Work out the finished part from the listing and answer in its coordinate system (mm). Coordinates: 2 decimals unless noted, no trailing zeros. Write each loop counter-clockwise with the first axis right and the second up, starting at its lowest first coordinate (ties: lowest second). Pieces come first, ordered by that corner, then holes. Notation, with made-up numbers: (45.25, 9) - (101.25, 9) arc R29 ccw to (101.25, 47) - close; hole circle Ø4 at (3, 52.25). An arc over 180 degrees is marked (long way). Use a Markdown table: item, result. Add a question column.
(1) Given pin 1 Ø7 at (x, y) = (-124.636, 30) entering from +Z; pin 2 Ø9 at (x, y) = (123.364, 90) entering from +Z, each flat-ended and moving along its own axis, determine where each tip first touches the part or whether it passes through.
(2) For a pull along Y with two mould halves and no side action, classify faces 1 (the face through (-32.157, -123.966, 151.736)), 2 (the face through (-120, 10, 150.75)), 3 (the face through (-120.94, 1.53, 151.74)) as released by +Y, released by -Y, zero draft, split by the parting line, or undercut.
(3) The part is cut by section B-B, the plane x = -108. Give the vertices of the cut face in (y, z), then the cut area to 3 significant figures.
(4) The part is cut by section C-C, the plane y = 83. Give the vertices of the cut face in (x, z).
(5) Find the intervals of material crossed by line 1 (X direction, y = -19, z = 152.15); line 2 (Y direction, x = 48, z = 151.7); line 3 (X direction, y = 89, z = 152.3), in increasing order. Write a range as from..to.
(6) The part is cut by section A-A, the plane y = 0. Give the vertices of the cut face in (x, z).
(7) The part is cut by section D-D, the plane z = 151.7. State how many separate pieces and enclosed holes the cut face has, then the cut area to 3 significant figures.
Autodesk Inventor part; units mm, degrees
ref_plane "YZ Plane" through (0, 0, 0) normal (1, 0, 0) x (0, 1, 0)
ref_plane "XZ Plane" through (0, 0, 0) normal (0, 1, 0) x (-1, 0, 0)
ref_plane "XY Plane" through (0, 0, 0) normal (0, 0, 1) x (1, 0, 0)
ref_plane "РабПлоскость1" through (-270.6167, -11.8042, 150.75) normal (0, 0, 1) x (1, 0, 0)
sketch "Эскиз1" plane through (-270.6167, -11.8042, 150.75) normal (0, 0, 1) x (1, 0, 0)
  circle A0 centre (393.9807, -108.1958) radius 4
  circle A1 centre (393.9807, -78.1958) radius 4
  circle A2 centre (393.9807, -48.1958) radius 4
  circle A3 centre (393.9807, -18.1958) radius 4
  circle A4 centre (393.9807, 11.8042) radius 4
  circle A5 centre (393.9807, 41.8042) radius 4
  circle A6 centre (393.9807, 71.8042) radius 4
  circle A7 centre (393.9807, 101.8042) radius 4
  circle A8 centre (393.9807, 131.8042) radius 4
  circle A9 centre (362.9807, -108.1958) radius 4
  circle A10 centre (362.9807, 131.8042) radius 4
  circle A11 centre (331.9807, -108.1958) radius 4
  circle A12 centre (331.9807, 131.8042) radius 4
  circle A13 centre (300.9807, -108.1958) radius 4
  circle A14 centre (300.9807, 131.8042) radius 4
  circle A15 centre (269.9807, -108.1958) radius 4
  circle A16 centre (269.9807, 131.8042) radius 4
  circle A17 centre (238.9807, -108.1958) radius 4
  circle A18 centre (238.9807, 131.8042) radius 4
  circle A19 centre (207.9807, -108.1958) radius 4
  circle A20 centre (207.9807, 131.8042) radius 4
  circle A21 centre (176.9807, -108.1958) radius 4
  circle A22 centre (176.9807, 131.8042) radius 4
  circle A23 centre (145.9807, -108.1958) radius 4
  circle A24 centre (145.9807, -78.1958) radius 4
  circle A25 centre (145.9807, -48.1958) radius 4
  circle A26 centre (145.9807, -18.1958) radius 4
  circle A27 centre (145.9807, 11.8042) radius 4
  circle A28 centre (145.9807, 41.8042) radius 4
  circle A29 centre (145.9807, 71.8042) radius 4
  circle A30 centre (145.9807, 101.8042) radius 4
  circle A31 centre (145.9807, 131.8042) radius 4
  line L0 (385.9807, 121.8042) -> (385.9807, -98.1958)
  line L1 (385.9807, -98.1958) -> (155.9807, -98.1958)
  line L2 (155.9807, -98.1958) -> (155.9807, 121.8042)
  line L3 (155.9807, 121.8042) -> (385.9807, 121.8042)
  arc A32 (137.9807, 141.8042) -> (135.9807, 139.8042) centre (137.9807, 139.8042) ccw
  line L4 (135.9807, 139.8042) -> (135.9807, -116.1958)
  arc A33 (135.9807, -116.1958) -> (137.9807, -118.1958) centre (137.9807, -116.1958) ccw
  line L5 (137.9807, -118.1958) -> (403.2527, -118.1958)
  arc A34 (403.2527, -118.1958) -> (405.2527, -116.1958) centre (403.2527, -116.1958) ccw
  line L6 (405.2527, -116.1958) -> (405.2527, 139.8042)
  arc A35 (405.2527, 139.8042) -> (403.2527, 141.8042) centre (403.2527, 139.8042) ccw
  line L7 (403.2527, 141.8042) -> (137.9807, 141.8042)
  point P0 (270.6167, 11.8042)
extrude "Выдавливание1" add sketch "Эскиз1" along normal blind 2
properties part number "Прокладка рубашки охлаждения"
Model answer:
| question | item | result |
|---|---|---|
| 1 | pin 1 | through |
| 1 | pin 2 | z = 152.75 |
| 2 | face 1 | undercut |
| 2 | face 2 | zero draft |
| 2 | face 3 | undercut |
| 3 | outline | (-130, 150.75) - (-110, 150.75) - (-110, 152.75) - (-130, 152.75) - close; (110, 150.75) - (130, 150.75) - (130, 152.75) - (110, 152.75) - close |
| 3 | area | 80.0 mm^2 |
| 4 | outline | (-134.64, 150.75) - (-114.64, 150.75) - (-114.64, 152.75) - (-134.64, 152.75) - close; (115.36, 150.75) - (134.64, 150.75) - (134.64, 152.75) - (115.36, 152.75) - close |
| 5 | line 1 | -134.64..-114.64, 115.36..134.64 |
| 5 | line 2 | -130..-110, 110..130 |
| 5 | line 3 | -134.64..-128.51, -120.76..-114.64, 115.36..119.49, 127.24..134.64 |
| 6 | outline | (-134.64, 150.75) - (-128.64, 150.75) - (-128.64, 152.75) - (-134.64, 152.75) - close; (-120.64, 150.75) - (-114.64, 150.75) - (-114.64, 152.75) - (-120.64, 152.75) - close; (115.36, 150.75) - (119.36, 150.75) - (119.36, 152.75) - (115.36, 152.75) - close; (127.36, 150.75) - (134.64, 150.75) - (134.64, 152.75) - (127.36, 152.75) - close |
| 7 | separate pieces | 1 |
| 7 | enclosed holes | 33 |
| 7 | area | 17,800 mm^2 |
